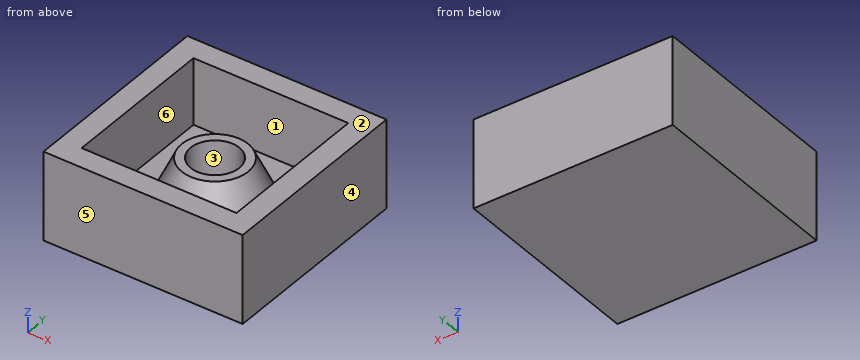
Autodesk Fusion 360 part; units mm, degrees
sketch "Sketch1" plane through (0, 0, 0) normal (0, 0, 1) x (1, 0, 0)
  line L0 (-22.5, 22.5) -> (22.5, 22.5)
  line L1 (22.5, 22.5) -> (22.5, -22.5)
  line L2 (22.5, -22.5) -> (-22.5, -22.5)
  line L3 (-22.5, -22.5) -> (-22.5, 22.5)
  line L4 (-22.5, 22.5) -> (22.5, -22.5) construction
  dimension "d1" = 45
extrude "Extrude1" add sketch "Sketch1" along normal blind 20
sketch "Sketch2" plane through (0, 0, 20) normal (0, 0, 1) x (-1, 0, 0)
  line L0 (22.5, 22.5) -> (-22.5, 22.5)
  line L1 (-22.5, 22.5) -> (-22.5, -22.5)
  line L2 (-22.5, -22.5) -> (22.5, -22.5)
  line L3 (22.5, -22.5) -> (22.5, 22.5)
  line L4 (-17.5, -17.5) -> (17.5, -17.5)
  line L5 (17.5, -17.5) -> (17.5, 17.5)
  line L6 (17.5, 17.5) -> (-17.5, 17.5)
  line L7 (-17.5, 17.5) -> (-17.5, -17.5)
  line L8 (-17.5, -17.5) -> (17.5, 17.5) construction
  line L9 (17.5, -17.5) -> (-17.5, 17.5) construction
  dimension "d4" = 5
  dimension "d5" = 5
extrude "Extrude2" cut sketch "Sketch2" against normal blind 15 contours L4 L5 L6 L7
sketch "Sketch3" plane through (0, 0, 0) normal (0, 1, 0) x (1, 0, 0)
  line L0 (22.5, -20) -> (22.5, 0)
  line L1 (22.5, 0) -> (-22.5, 0)
  line L2 (-22.5, 0) -> (-22.5, -20)
  line L3 (-22.5, -20) -> (-17.5, -20)
  line L4 (-17.5, -20) -> (-17.5, -5)
  line L5 (-17.5, -5) -> (17.5, -5)
  line L6 (17.5, -5) -> (17.5, -20)
  line L7 (17.5, -20) -> (22.5, -20)
  line L8 (-7.5, -15) -> (7.5, -15)
  line L9 (0, -15) -> (0, -5) construction
  line L10 (-7.5, -15) -> (-12.1631, -5)
  line L11 (7.5, -15) -> (12.1631, -5)
  line L12 (-5.5, -15) -> (5.5, -15)
  line L13 (5.5, -15) -> (5.5, -5)
  line L14 (5.5, -5) -> (-5.5, -5)
  line L15 (-5.5, -5) -> (-5.5, -15)
  dimension "d8" = 15
  dimension "d9" = 65
  dimension "d10" = 65
  dimension "d11" = 11
  dimension "d12" = 10
revolve "Revolve1" add sketch "Sketch3" angle 360 about axis through (0, 0, 15) along (0, 0, -1) contours L5 L8 L10 L15
Geometry check sheet. Reference: the model listing, model coordinates, mm. Face numbers are marked on the shaded views. A direction names the side the tool comes from. Coordinates: 2 decimals unless noted, no trailing zeros. Loops run counter-clockwise (first coordinate to the right, second up) from the corner with the lowest first, then second, coordinate; pieces in that order, holes last.
Item 1: Sectioned sample at B-B, the plane z = 13.25. Record the boundary of the cut face in (x, y).
Item 2: Release check for a two-part mould opening along Y. For the marked faces 3, 4, 5 and 6 record: released by +Y, released by -Y, zero draft, split by the parting line, or undercut.
Item 3: Go/stop test with flat-tipped pins: pin 1 Ø16.5 at (x, y) = (0.5, 0.5) entering from +Z; pin 2 Ø2 at (x, y) = (13.5, -13.5) entering from +Z. Record where each tip stops, or that it passes through.
Item 4: Thickness scan on line 1 (X direction, y = -13.5, z = 13.5); line 2 (Y direction, x = 0, z = 10). Record the ranges inside material, lowest first.
Item 5: Access from +Z, -Z, +X, -X, +Y, -Y to the whole of each face (thin tool, end or side, straight path). Record for the marked faces 1 and 2.
Item 6: Sectioned sample at A-A, the plane x = 0. Record the boundary of the cut face in (y, z).
Item 7: Sectioned sample at C-C, the plane y = -14. Record the boundary of the cut face in (x, z), then the cut area to 3 significant figures.
Check result:
1. outline: (-22.5, -22.5) - (22.5, -22.5) - (22.5, 22.5) - (-22.5, 22.5) - close; circle Ø16.63 at (0, 0); hole (-17.5, -17.5) - (17.5, -17.5) - (17.5, 17.5) - (-17.5, 17.5) - close; hole circle Ø11 at (0, 0)
2. face 3: undercut
2. face 4: zero draft
2. face 5: released by -Y
2. face 6: undercut
3. pin 1: stops at z = 15
3. pin 2: stops at z = 5
4. line 1: x = -22.5 to -17.5, 17.5 to 22.5
4. line 2: y = -22.5 to -17.5, -9.83 to -5.5, 5.5 to 9.83, 17.5 to 22.5
5. face 1: +Z
5. face 2: +Z, +X, -X, +Y, -Y
6. outline: (-22.5, 0) - (22.5, 0) - (22.5, 20) - (17.5, 20) - (17.5, 5) - (12.16, 5) - (7.5, 15) - (5.5, 15) - (5.5, 5) - (-5.5, 5) - (-5.5, 15) - (-7.5, 15) - (-12.16, 5) - (-17.5, 5) - (-17.5, 20) - (-22.5, 20) - close
7. outline: (-22.5, 0) - (22.5, 0) - (22.5, 20) - (17.5, 20) - (17.5, 5) - (-17.5, 5) - (-17.5, 20) - (-22.5, 20) - close
7. area: 375 mm2
